Verification items for the finished model (mm, model axes). Face numbers are marked on the shaded views. Give positions to 0.01 mm unless a question says otherwise; leave off trailing zeros. Loops run counter-clockwise (first coordinate to the right, second up) from the corner with the lowest first, then second, coordinate; pieces in that order, holes last. Notation, with made-up numbers: (54.25, 48) - (83.25, 48) arc R22 ccw to (83.25, 65) - close; hole circle Ø2 at (-29, 13). An arc over 180 degrees is marked (long way). One line per question, with ' | ' between items. Start each with the question number.
1. Thickness scan on line 1 along X through (y, z) = (-2.5, 13); line 2 along X through (y, z) = (-1.25, 9.5); line 3 along Z through (x, y) = (-20.5, -3.75). Record the ranges inside material, lowest first. Write a range as from..to.
2. Mould release check, pull along X, two halves, no side actions. Record for the marked faces 1, 2 and 3: +X half, -X half, draft (parallel to the pull), parting line (faces both ways), or undercut.
3. Depth check by flat-ended pin: pin 1 Ø6 at (x, y) = (-25, -9) entering from -Z; pin 2 Ø4 at (x, y) = (1, 2) entering from -Z; pin 3 Ø5.5 at (x, y) = (-21.5, 0.5) entering from -Z. Enter the tip coordinate at first touch or a pass-through.
4. Section check D-D, the plane x = 20. Enter the section's corners in (y, z), then the cut area to 3 significant figures.
5. Section check B-B, the plane y = 2.75. Enter the section's corners in (x, z).
6. Section check C-C, the plane z = 8.5. Enter the section's corners in (x, y), then the cut area to 3 significant figures.
7. Section check A-A, the plane z = 12.5. Enter the section's corners in (x, y).
from build123d import *

# Parameters (mm, degrees)
SKETCH_1_W          = 70
SKETCH_1_H          = 30
EXTRUDE_1_DEPTH     = 15.75
CUT_EXTRUDE_1_DEPTH = 30
SKETCH_4_W          = 70
SKETCH_4_H          = 4
CUT_EXTRUDE_2_DEPTH = 30
SKETCH_6_W          = 5
SKETCH_6_H          = 10
CUT_EXTRUDE_3_DEPTH = 10


with BuildPart() as part:
    # 草图1 → 凸台-拉伸1 (new body)
    with BuildSketch(Plane.XY):
        Rectangle(SKETCH_1_W, SKETCH_1_H)
    extrude(amount=EXTRUDE_1_DEPTH)

    # 草图3 → 切除-拉伸1 (cut)
    with BuildSketch(Plane(origin=(0, 15, 0), x_dir=(1, 0, 0), z_dir=(0, 1, 0))):
        with BuildLine():
            ThreePointArc((-32.25, 0), (-21.5, -10.75), (-10.75, 0))
            Line((-10.75, 0), (-32.25, 0))
        make_face()
        with BuildLine():
            Line((10.75, 0), (-10.75, 0))
            ThreePointArc((-10.75, 0), (0, -10.75), (10.75, 0))
        make_face()
        with BuildLine():
            Line((32.25, 0), (10.75, 0))
            ThreePointArc((10.75, 0), (21.5, -10.75), (32.25, 0))
        make_face()
    extrude(amount=-CUT_EXTRUDE_1_DEPTH, mode=Mode.SUBTRACT)

    # 草图4 → 切除-拉伸2 (cut)
    with BuildSketch(Plane(origin=(0, 15, 0), x_dir=(1, 0, 0), z_dir=(0, 1, 0))):
        with Locations((0, -2)):
            Rectangle(SKETCH_4_W, SKETCH_4_H)
    extrude(amount=-CUT_EXTRUDE_2_DEPTH, mode=Mode.SUBTRACT)

    # 草图6 → 切除-拉伸3 (cut)
    with BuildSketch(Plane(origin=(0, 0, 4), x_dir=(-1, 0, 0), z_dir=(0, 0, -1))):
        with Locations((21.5, 0)):
            Rectangle(SKETCH_6_W, SKETCH_6_H)
        Rectangle(SKETCH_6_W, SKETCH_6_H)
        with Locations((-21.5, 0)):
            Rectangle(SKETCH_6_W, SKETCH_6_H)
    extrude(amount=-CUT_EXTRUDE_3_DEPTH, mode=Mode.SUBTRACT)


solid = part.part
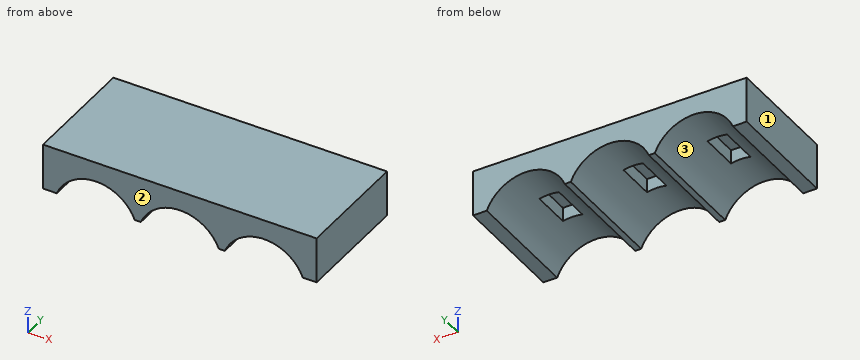
Results list:
1) line 1: -35..-24, -19..-2.5, 2.5..19, 24..35 | line 2: -35..-26.53, -16.47..-5.03, 5.03..16.47, 26.53..35 | line 3: 14..15.75
2) face 1: -X half | face 2: draft | face 3: undercut
3) pin 1: z = 8.56 | pin 2: z = 10.32 | pin 3: z = 10.39
4) outline: (-15, 10.64) - (-5, 10.64) - (-5, 14) - (5, 14) - (5, 10.64) - (15, 10.64) - (15, 15.75) - (-15, 15.75) - close | area: 120 mm²
5) outline: (-35, 4) - (-31.48, 4) arc R10.75 cw to (-24, 10.46) - (-24, 14) - (-19, 14) - (-19, 10.46) arc R10.75 cw to (-11.52, 4) - (-9.98, 4) arc R10.75 cw to (-2.5, 10.46) - (-2.5, 14) - (2.5, 14) - (2.5, 10.46) arc R10.75 cw to (9.98, 4) - (11.52, 4) arc R10.75 cw to (19, 10.46) - (19, 14) - (24, 14) - (24, 10.46) arc R10.75 cw to (31.48, 4) - (35, 4) - (35, 15.75) - (-35, 15.75) - close
6) outline: (-35, -15) - (-28.08, -15) - (-28.08, 15) - (-35, 15) - close; (-14.92, -15) - (-6.58, -15) - (-6.58, 15) - (-14.92, 15) - close; (6.58, -15) - (14.92, -15) - (14.92, 15) - (6.58, 15) - close; (28.08, -15) - (35, -15) - (35, 15) - (28.08, 15) - close | area: 915 mm²
7) outline: (-35, -15) - (35, -15) - (35, 15) - (-35, 15) - close; hole (-24, -5) - (-19, -5) - (-19, 5) - (-24, 5) - close; hole (-2.5, -5) - (2.5, -5) - (2.5, 5) - (-2.5, 5) - close; hole (19, -5) - (24, -5) - (24, 5) - (19, 5) - close
